Work out the finished part from the listing and answer in its coordinate system (mm). A direction names the side the tool comes from. Round coordinates to 2 decimals unless told otherwise and drop trailing zeros. Loops run counter-clockwise (first coordinate to the right, second up) from the corner with the lowest first, then second, coordinate; pieces in that order, holes last. Notation, with made-up numbers: M -17,56 L 22,56 A15 cw 22,85 Z; hole C 35.5,-1.5 d1. An arc over 180 degrees is marked long. One line per item, written item: value.
```python
from build123d import *

# Parameters (mm, degrees)
BOSS_EXTRUDE1_DEPTH = 18.59
CUT_EXTRUDE2_DEPTH  = 1238.071375507
SKETCH4_R           = 5.207
BOSS_EXTRUDE3_DEPTH = 23.2


with BuildPart() as part:
    # Sketch2 → Boss-Extrude1 (new body)
    with BuildSketch(Plane.XY):
        Polygon((0, 0), (1200, 0), (1200, -18.59), (800, -300), (400, -300), (0, -18.59), align=None)
    extrude(amount=BOSS_EXTRUDE1_DEPTH)

    # Sketch3 → Cut-Extrude2 (cut, through all)
    with BuildSketch(Plane.XY.offset(18.59)):
        Polygon((32.308203874, -18.59), (400, -281.41), (587.859378773, -18.59), align=None)
        Polygon((600.156298082, -33.792330813), (423.163293339, -281.41), (777.149302825, -281.41), align=None)
        Polygon((800, -281.41), (1167.691796126, -18.59), (612.140621227, -18.59), align=None)
    extrude(amount=-CUT_EXTRUDE2_DEPTH, mode=Mode.SUBTRACT)

    # Sketch4 → Boss-Extrude3 (add)
    with BuildSketch(Plane(origin=(0, 0, 0), x_dir=(-1, 0, 0), z_dir=(0, 0, -1))):
        with Locations((-1190.705, -9.295)):
            Circle(SKETCH4_R)
        with Locations((-600.156298082, -9.295)):
            Circle(SKETCH4_R)
        with Locations((-9.295, -9.295)):
            Circle(SKETCH4_R)
        with Locations((-790.705, -290.705)):
            Circle(SKETCH4_R)
        with Locations((-409.295, -290.705)):
            Circle(SKETCH4_R)
    extrude(amount=-BOSS_EXTRUDE3_DEPTH)


solid = part.part
```
1) For faces 1 (the face through (894, -18.59, 9)), 2 (the face through (0, -9, 9)), determine the directions among +Z, -Z, +X, -X, +Y, -Y from which every point of the face is accessible in a straight line to the end or side of a thin tool.
Check values:
face 1: +Z, -Z
face 2: +Z, -Z, -X, +Y, -Y
2) The mould has two halves that part along Y. Classify faces 3 (the face through (981.27, -151.84, 9.43)), 4 (the face through (213.58, -148.16, 9.43)), 5 (the face through (1002.8, -157.325, 9.165)), 6 (the face through (1200, -9, 9)): +Y half, -Y half, draft (parallel to the pull), parting line (faces both ways), or undercut.
Check values:
face 3: undercut
face 4: undercut
face 5: -Y half
face 6: draft
3) Find section C-C (y = -170). Give the vertices of the cut face in (x, z), then the cut area to 3 significant figures.
Check values:
outline: M 215.22,0 L 244.13,0 L 244.13,18.59 L 215.22,18.59 Z; M 479.63,0 L 502.8,0 L 502.8,18.59 L 479.63,18.59 Z; M 697.52,0 L 720.37,0 L 720.37,18.59 L 697.52,18.59 Z; M 955.87,0 L 984.78,0 L 984.78,18.59 L 955.87,18.59 Z
area: 1,930 mm2
4) Each of these flat-tipped pins is pushed along its axis until it touches: pin 1 (6 mm diameter, centred on x = 1020.5, z = 16.5, fed in from -Y); pin 2 (8 mm diameter, centred on x = 462.5, z = 20.5, fed in from +Y); pin 3 (12 mm diameter, centred on y = -262, z = 19, fed in from +X). Where does it stop, or does it pass through?
Check values:
pin 1: y = -146.98
pin 2: y = 0
pin 3: x = 862.52
5) Find section A-A (z = 7.25). Give the vertices of the cut face in (x, y), then the cut area to 3 significant figures.
Check values:
outline: M 0,-18.59 L 400,-300 L 800,-300 L 1200,-18.59 L 1200,0 L 0,0 Z; hole M 32.31,-18.59 L 400,-281.41 L 587.86,-18.59 Z; hole M 423.16,-281.41 L 777.15,-281.41 L 600.16,-33.79 Z; hole M 612.14,-18.59 L 800,-281.41 L 1167.69,-18.59 Z
area: 57,600 mm2
6) Find section B-B (x = 85). Give the vertices of the cut face in (y, z), then the cut area to 3 significant figures.
Check values:
outline: M -78.39,0 L -56.25,0 L -56.25,18.59 L -78.39,18.59 Z; M -18.59,0 L 0,0 L 0,18.59 L -18.59,18.59 Z
area: 757 mm2
7) Find the intervals of material crossed by probe 1 along X at (y, z) = (-162.5, 18); probe 2 along X at (y, z) = (-133.5, 5.25); probe 3 along Y at (x, z) = (510.5, 3.75), in increasing order. Write a range as from..to.
Check values:
probe 1: 204.56..233.64, 484.99..508.16, 692.15..715.01, 966.36..995.44
probe 2: 163.33..193.07, 505.72..528.89, 671.43..694.28, 1006.93..1036.67
probe 3: -300..-281.41, -159.22..-126.82, -18.59..0
8) Find section D-D (x = 734). Give the vertices of the cut face in (y, z).
Check values:
outline: M -300,0 L -281.41,0 L -281.41,18.59 L -300,18.59 Z; M -221.04,0 L -189.07,0 L -189.07,18.59 L -221.04,18.59 Z; M -18.59,0 L 0,0 L 0,18.59 L -18.59,18.59 Z
